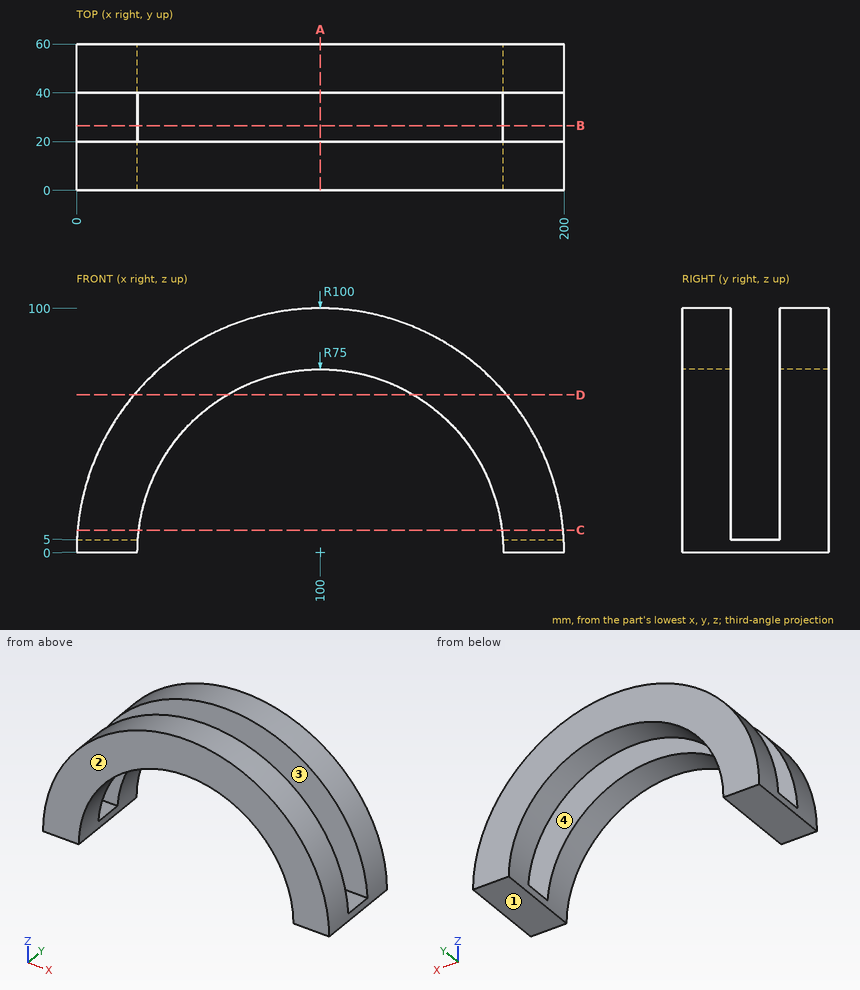
Geometry check sheet. Reference: drawing and pictorial views, mm from the part's lowest x, y, z. Coordinates: 2 decimals unless noted, no trailing zeros. Write each loop counter-clockwise with the first axis right and the second up, starting at its lowest first coordinate (ties: lowest second). Pieces come first, ordered by that corner, then holes. Notation, with made-up numbers: M 12,57.25 L 68,57.25 A21 cw 68,66.25 Z; hole C 49.5,-20.5 d6. An arc over 180 degrees is marked long. Write item = value, one per line. Start each with the question number.
1. Mould release check, pull along Y, two halves, no side actions. Record for the marked faces 1, 2, 3 and 4: pulls with the +Y half, pulls with the -Y half, needs draft (parallel to the pull), parting line crosses it, or undercut.
2. Sectioned sample at C-C (z = 9). Record the cut outline in (x, y).
3. Sectioned sample at D-D (z = 64.5). Record the cut outline in (x, y), then the cut area to 3 significant figures.
4. Sectioned sample at B-B (y = 26.5). Record the cut outline in (x, z), then the cut area to 3 significant figures.
5. Thickness scan on probe 1 along Y at (x, z) = (31, 38); probe 2 along X at (y, z) = (14, 68.5); probe 3 along Z at (x, y) = (19.5, 28). Record the ranges inside material, lowest first.
6. Go/stop test with flat-tipped pins: pin 1 (4 mm diameter, centred on y = 18, z = 38.5, fed in from -X); pin 2 (10 mm diameter, centred on x = 192, y = 27.5, fed in from +Z); pin 3 (4 mm diameter, centred on x = 94, y = 23, fed in from +Z); pin 4 (5 mm diameter, centred on x = 156, y = 44, fed in from -Z). Record where each tip stops, or that it passes through.
7. Sectioned sample at A-A (x = 100). Record the cut outline in (y, z), then the cut area to 3 significant figures.
The answers:
q1.face_1 = needs draft
q1.face_2 = pulls with the -Y half
q1.face_3 = undercut
q1.face_4 = undercut
q2.outline = M 0.41,0 L 25.54,0 L 25.54,20 L 0.41,20 Z; M 0.41,40 L 25.54,40 L 25.54,60 L 0.41,60 Z; M 174.46,0 L 199.59,0 L 199.59,20 L 174.46,20 Z; M 174.46,40 L 199.59,40 L 199.59,60 L 174.46,60 Z
q3.outline = M 23.58,0 L 61.73,0 L 61.73,20 L 23.58,20 Z; M 23.58,40 L 61.73,40 L 61.73,60 L 23.58,60 Z; M 138.27,0 L 176.42,0 L 176.42,20 L 138.27,20 Z; M 138.27,40 L 176.42,40 L 176.42,60 L 138.27,60 Z
q3.area = 3,050 mm²
q4.outline = M 0,0 L 25,0 A75 cw 25.17,5 L 0.13,5 A100 ccw Z; M 174.83,5 A75 cw 175,0 L 200,0 A100 ccw 199.87,5 Z
q4.area = 250 mm²
q5.probe_1 = 0 to 20, 40 to 60
q5.probe_2 = 27.15 to 69.46, 130.54 to 172.85
q5.probe_3 = 0 to 5
q6.pin_1 = 6.9
q6.pin_2 = 5
q6.pin_3 = through
q6.pin_4 = 46.93
q7.outline = M 0,75 L 20,75 L 20,100 L 0,100 Z; M 40,75 L 60,75 L 60,100 L 40,100 Z
q7.area = 1,000 mm²
